```python
from build123d import *

# Parameters (mm, degrees)
BOSS_EXTRUDE1_DEPTH = 4
SKETCH2_R           = 0.35
BOSS_EXTRUDE2_DEPTH = 3.41


with BuildPart() as part:
    # Sketch1 → Boss-Extrude1 (new body)
    with BuildSketch(Plane(origin=(0, 0, 0), x_dir=(1, 0, 0), z_dir=(0, 1, 0))):
        Polygon((-1.016, -1.016), (0.254, -2.286), (2.286, -2.286), (3.556, -1.016), (3.556, 1.016), (-1.016, 1.016), align=None)
    extrude(amount=BOSS_EXTRUDE1_DEPTH)

    # Sketch2 → Boss-Extrude2 (add)
    with BuildSketch(Plane.XZ):
        Circle(SKETCH2_R)
        with Locations((2.54, 0)):
            Circle(SKETCH2_R)
        with Locations((1.27, 1.2755783)):
            Circle(SKETCH2_R)
    extrude(amount=BOSS_EXTRUDE2_DEPTH)


solid = part.part
```
Build history of the part. All positions in model axes, mm. A direction names the side the tool comes from. Round coordinates to 2 decimals unless told otherwise and drop trailing zeros. Order: outer loops, then holes, each group sorted by start corner. A loop starts at its lowest first (then second) coordinate and runs counter-clockwise, first axis right, second up. Notation, with made-up numbers: (85, -22) - (135, -22) arc R32 ccw to (135, 11) - close; hole circle Ø10 at (-28.75, -37). An arc over 180 degrees is marked (long way). Use a Markdown table: item, result.
1) Flat gauge pins, fed straight in: pin 1 Ø1 at (x, z) = (2, 2) entering from -Y; pin 2 Ø1.5 at (x, y) = (2.5, 0) entering from +Z. Where does each tip first touch, or does it go through?
Recorded:
| item | result |
|---|---|
| pin 1 | stops at y = 0 |
| pin 2 | stops at z = 2.29 |
2) Saw through at D-D on x = 1.27. Write the cut outline in (y, z).
Recorded:
| item | result |
|---|---|
| outline | (-3.41, 0.93) - (0, 0.93) - (0, -1.02) - (4, -1.02) - (4, 2.29) - (0, 2.29) - (0, 1.63) - (-3.41, 1.63) - close |
3) Saw through at B-B on x = 0. Write the cut outline in (y, z).
Recorded:
| item | result |
|---|---|
| outline | (-3.41, -0.35) - (0, -0.35) - (0, -1.02) - (4, -1.02) - (4, 2.03) - (0, 2.03) - (0, 0.35) - (-3.41, 0.35) - close |
4) Saw through at C-C on y = 3. Write the cut outline in (x, z).
Recorded:
| item | result |
|---|---|
| outline | (-1.02, -1.02) - (3.56, -1.02) - (3.56, 1.02) - (2.29, 2.29) - (0.25, 2.29) - (-1.02, 1.02) - close |
5) Saw through at A-A on z = 0. Write the cut outline in (x, y), and give its area (3 significant figures).
Recorded:
| item | result |
|---|---|
| outline | (-1.02, 0) - (-0.35, 0) - (-0.35, -3.41) - (0.35, -3.41) - (0.35, 0) - (2.19, 0) - (2.19, -3.41) - (2.89, -3.41) - (2.89, 0) - (3.56, 0) - (3.56, 4) - (-1.02, 4) - close |
| area | 23.1 mm² |
6) Wall check: L1, parallel to Y at x = 3, z = 0.7; L2, parallel to X at y = -2, z = 1.3; L3, parallel to X at y = -0.25, z = -0.25. Give the ranges that are in metal, low to high.
Recorded:
| item | result |
|---|---|
| L1 | y = 0 to 4 |
| L2 | x = 0.92 to 1.62 |
| L3 | x = -0.24 to 0.24, 2.3 to 2.78 |
7) Tool access for faces 1 (the face through (1.2, 0, 0.6)), 2 (the face through (1, 2, 2.286)): list every direction of +Z, -Z, +X, -X, +Y, -Y with a clear straight run to the whole face (end or side of a thin tool).
Recorded:
| item | result |
|---|---|
| face 1 | -Y |
| face 2 | +Z, +X, -X, +Y, -Y |
